```python
from build123d import *

# Parameters (mm, degrees)
BOSS_EXTRUDE1_DEPTH = 25.4
FILLET1_R           = 12.7
CUT_EXTRUDE1_REACH  = 67.579
SKETCH2_R           = 2.5
CUT_EXTRUDE2_REACH  = 70.586
SKETCH3_R           = 2.5


with BuildPart() as part:
    # Sketch1 → Boss-Extrude1 (new body)
    with BuildSketch(Plane(origin=(0, 0, 0), x_dir=(1, 0, 0), z_dir=(0, 1, 0))):
        Polygon((10.375, 15.95), (-15.025, 15.95), (-15.025, -9.45), (10.375, -9.45), (10.375, -17.45), (-23.025, -17.45), (-23.025, -12.25), (-48.425, -12.25), (-48.425, -4.25), (-23.025, -4.25), (-23.025, 10.75), (-48.425, 10.75), (-48.425, 18.75), (-23.025, 18.75), (-23.025, 23.95), (10.375, 23.95), align=None)
    extrude(amount=BOSS_EXTRUDE1_DEPTH)

    # Fillet1
    fillet1_edges = [part.edges().sort_by_distance(p)[0] for p in [
        (-48.425, 25.4, -14.75),
        (-48.425, 0, -14.75),
        (-48.425, 0, 8.25),
        (-48.425, 25.4, 8.25),
    ]]
    fillet(fillet1_edges, radius=FILLET1_R - 0.0001)  # a hair under: the kernel refuses the full size

    # Cut-Extrude1: up to this face of the body (flat: up to its plane)
    cut_extrude1_end = Plane(part.part.faces().sort_by_distance((-34.539475021, 12.7, -18.75))[0])
    # Sketch2 → Cut-Extrude1 (cut, up to the picked face)
    with BuildSketch(Plane.XY.offset(12.25), mode=Mode.PRIVATE) as cut_extrude1_sk1:
        with Locations((-35.725, 12.7)):
            Circle(SKETCH2_R)
    cut_extrude1_tool1 = split(extrude(cut_extrude1_sk1.sketch, amount=-CUT_EXTRUDE1_REACH, mode=Mode.PRIVATE), bisect_by=cut_extrude1_end, keep=Keep.BOTH, mode=Mode.PRIVATE)
    add(cut_extrude1_tool1.solids().sort_by(Axis((-35.725, 12.7, 12.25), (0, 0, -1)))[0], mode=Mode.SUBTRACT)

    # Cut-Extrude2: up to this face of the body (flat: up to its plane)
    cut_extrude2_end = Plane(part.part.faces().sort_by_distance((-6.325, 12.7, -23.95))[0])
    # Sketch3 → Cut-Extrude2 (cut, up to the picked face)
    with BuildSketch(Plane.XY.offset(17.45), mode=Mode.PRIVATE) as cut_extrude2_sk1:
        with Locations((-2.125, 12.7)):
            Circle(SKETCH3_R)
    cut_extrude2_tool1 = split(extrude(cut_extrude2_sk1.sketch, amount=-CUT_EXTRUDE2_REACH, mode=Mode.PRIVATE), bisect_by=cut_extrude2_end, keep=Keep.BOTH, mode=Mode.PRIVATE)
    add(cut_extrude2_tool1.solids().sort_by(Axis((-2.125, 12.7, 17.45), (0, 0, -1)))[0], mode=Mode.SUBTRACT)


solid = part.part
```
Input: part model. Units: mm. Frame: model coordinates. A direction names the side the tool comes from. Coordinates: 2 decimals unless noted, no trailing zeros. Loops run counter-clockwise (first coordinate to the right, second up) from the corner with the lowest first, then second, coordinate; pieces in that order, holes last. Notation, with made-up numbers: M 57,31.25 L 92,31.25 A25 ccw 92,51.25 Z; hole C 24.25,10.25 d6. An arc over 180 degrees is marked long. Answer in a Markdown table with one row per item.
1. Section C-C, the plane y = 11. Count the separate pieces of the cut face and the enclosed holes in it, then the cut area to 3 significant figures.
Response:
| item | result |
|---|---|
| separate pieces | 5 |
| enclosed holes | 0 |
| area | 1,020 mm2 |
2. Material intervals for line 1 (X direction, y = 12.75, z = -18) (1 decimal); line 2 (Z direction, x = -41.5, y = 15.5); line 3 (Z direction, x = 1, y = 8.5), sorted ascending.
Response:
| item | result |
|---|---|
| line 1 | x = -48.4 to -38.2, -33.2 to -4.6, 0.4 to 10.4 |
| line 2 | z = -18.75 to -10.75, 4.25 to 12.25 |
| line 3 | z = -23.95 to -15.95, 9.45 to 17.45 |
3. First-contact query: pin 1 (8 mm diameter, centred on x = -35.725, y = 12.7, fed in from +Z); pin 2 (7.5 mm diameter, centred on y = 17.5, z = -7.5, fed in from +X) (3 decimals); pin 3 (1.6 mm diameter, centred on y = 15, z = 15.5, fed in from -X) (3 decimals). Flat tips, straight axial feed; report the tip coordinate or a pass-through.
Response:
| item | result |
|---|---|
| pin 1 | stops at z = 12.25 |
| pin 2 | stops at x = -15.025 |
| pin 3 | stops at x = -23.025 |
4. Draft query along X for faces 6 (the flat face through (-6, 13, 17.45)), 7 (the flat face through (10.375, 13, -20)), 8 (the flat face through (-23.025, 13, -21)), 9 (the cylindrical face through (-33.34, 13.45, 8.31)). Return one class per face: pulls with the +X half, pulls with the -X half, needs draft (parallel to the pull), parting line crosses it, or undercut.
Response:
| item | result |
|---|---|
| face 6 | needs draft |
| face 7 | pulls with the +X half |
| face 8 | pulls with the -X half |
| face 9 | undercut |
5. Section B-B, the plane x = -12.5. Output: boundary loops of the cut face in (y, z), then the cut area to 3 significant figures.
Response:
| item | result |
|---|---|
| outline | M 0,-23.95 L 25.4,-23.95 L 25.4,-15.95 L 0,-15.95 Z; M 0,9.45 L 25.4,9.45 L 25.4,17.45 L 0,17.45 Z |
| area | 406 mm2 |
6. Section D-D, the plane x = -2. Output: boundary loops of the cut face in (y, z), then the cut area to 4 significant figures.
Response:
| item | result |
|---|---|
| outline | M 0,-23.95 L 10.2,-23.95 L 10.2,-15.95 L 0,-15.95 Z; M 0,9.45 L 10.2,9.45 L 10.2,17.45 L 0,17.45 Z; M 15.2,-23.95 L 25.4,-23.95 L 25.4,-15.95 L 15.2,-15.95 Z; M 15.2,9.45 L 25.4,9.45 L 25.4,17.45 L 15.2,17.45 Z |
| area | 326.5 mm2 |
7. Reachability of faces 1 (the flat face through (-33, 13, 4.25)), 2 (the flat face through (-5, 13, 9.45)), 3 (the flat face through (-33, 13, 12.25)), 4 (the flat face through (-33, 13, -18.75)), 5 (the cylindrical face through (-2.45, 15.18, 13.51)) from +Z, -Z, +X, -X, +Y, -Y: full face, straight path, thin tool, end or side. Return the list, or none.
Response:
| item | result |
|---|---|
| face 1 | -X, +Y, -Y |
| face 2 | +X, +Y, -Y |
| face 3 | +Z, -X, +Y, -Y |
| face 4 | -Z, -X, +Y, -Y |
| face 5 | +Z, -Z |
